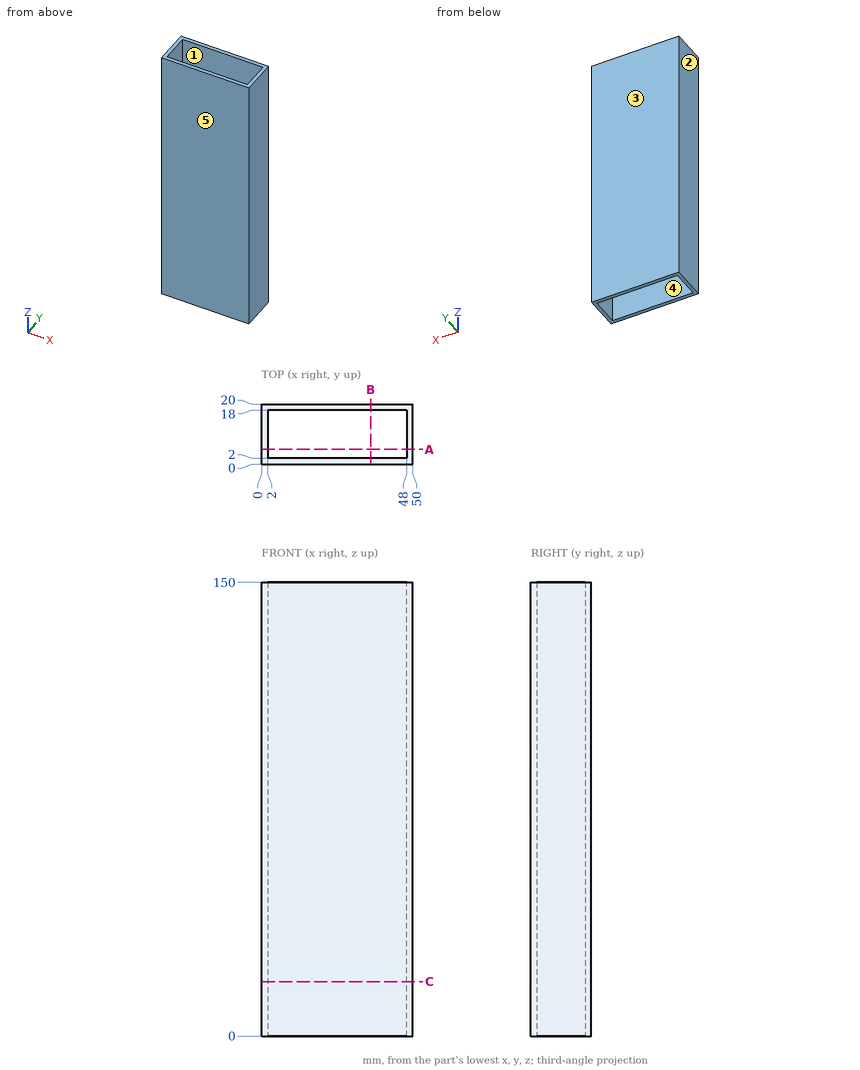
Drawing for the job (mm, zero at the part's lowest x, y, z). A direction names the side the tool comes from. Round coordinates to 2 decimals unless told otherwise and drop trailing zeros. Write each loop counter-clockwise with the first axis right and the second up, starting at its lowest first coordinate (ties: lowest second). Pieces come first, ordered by that corner, then holes. Notation, with made-up numbers: M -25.5,25.5 L 2.5,25.5 A17 ccw 2.5,39.5 Z; hole C 29.5,-22 d8. An arc over 180 degrees is marked long. Answer in a Markdown table with one row per item.
1. Which spindle directions (+Z, -Z, +X, -X, +Y, -Y) get a long thin tool onto all of the face, cutting with end or side? Do the marked faces 4 and 5. Say none if no direction does.
Geometry check:
| item | result |
|---|---|
| face 4 | +Z, -Z |
| face 5 | +Z, -Z, +X, -X, -Y |
2. Mould opens along Y. For the marked faces 1, 2 and 3 say: +Y half, -Y half, draft (parallel to the pull), parting line (faces both ways), or undercut.
Geometry check:
| item | result |
|---|---|
| face 1 | undercut |
| face 2 | draft |
| face 3 | +Y half |
3. Probe L1, parallel to Y at x = 47, z = 118.5; L2, parallel to X at y = 13.5, z = 55. List the from-to ranges inside material, lowest first. Write a range as [from, to].
Geometry check:
| item | result |
|---|---|
| L1 | [0, 2], [18, 20] |
| L2 | [0, 2], [48, 50] |
4. Saw through at A-A (y = 5). List the corners of the cut face in (x, z), and give its area (3 significant figures).
Geometry check:
| item | result |
|---|---|
| outline | M 0,0 L 2,0 L 2,150 L 0,150 Z; M 48,0 L 50,0 L 50,150 L 48,150 Z |
| area | 600 mm2 |
5. Saw through at C-C (z = 18). List the corners of the cut face in (x, y), and give its area (3 significant figures).
Geometry check:
| item | result |
|---|---|
| outline | M 0,0 L 50,0 L 50,20 L 0,20 Z; hole M 2,2 L 48,2 L 48,18 L 2,18 Z |
| area | 264 mm2 |
6. Saw through at B-B (x = 36). List the corners of the cut face in (y, z), and give its area (3 significant figures).
Geometry check:
| item | result |
|---|---|
| outline | M 0,0 L 2,0 L 2,150 L 0,150 Z; M 18,0 L 20,0 L 20,150 L 18,150 Z |
| area | 600 mm2 |
7. Flat gauge pin, fed straight in: P1, Ø1.5, axis at x = 19.5, y = 4.5, coming from the -Z side. Where does the tip first touch, or does it go through?
Geometry check:
| item | result |
|---|---|
| P1 | through |
